from build123d import *

# Parameters (mm, degrees)
PAD005_DEPTH    = 50
SKETCH012_R     = 2.1
POCKET004_DEPTH = 50.001
POCKET005_DEPTH = 8
SKETCH014_W     = 7.2
SKETCH014_H     = 3.4
POCKET006_DEPTH = 8.85
SKETCH015_R     = 1.45
POCKET007_DEPTH = 21.801
FILLET012_R     = 3
FILLET013_R     = 3
FILLET015_R     = 1


with BuildPart() as part:
    # Sketch010 → Pad005 (new body)
    with BuildSketch(Plane.XZ):
        Polygon((-9.9, -11.8), (9.9, -11.8), (9.9, 0), (19.1, 0), (19.1, 10), (-19.1, 10), (-19.1, 0), (-9.9, 0), align=None)
    extrude(amount=PAD005_DEPTH)

    # Sketch012 → Pocket004 (cut, through all)
    with BuildSketch(Plane.XZ):
        with Locations((0, -7)):
            Circle(SKETCH012_R)
    extrude(amount=POCKET004_DEPTH, mode=Mode.SUBTRACT)

    # Sketch013 → Pocket005 (cut, symmetric)
    with BuildSketch(Plane.YZ):
        with BuildLine():
            Line((-24.861402, 6.200002), (-36.703512, -3.006758))
            ThreePointArc((-45.296488, 8.045878), (-46.526318, -1.776928), (-36.703512, -3.006758))
            Line((-42.783017, 10), (-45.296488, 8.045878))
            Line((0, 10), (-42.783017, 10))
            Line((0.003511, 6.200002), (0, 10))
            Line((-24.861402, 6.200002), (0.003511, 6.200002))
        make_face()
        with BuildLine():
            ThreePointArc((-43.455136, 5.677456), (-44.157896, 0.064424), (-38.544864, -0.638336))
            Line((-38.544864, -0.638336), (-29.749115, 6.200002))
            Line((-42.783017, 6.200002), (-29.749115, 6.200002))
            Line((-43.455136, 5.677456), (-42.783017, 6.200002))
        make_face(mode=Mode.SUBTRACT)
    extrude(amount=POCKET005_DEPTH, both=True, mode=Mode.SUBTRACT)

    # Sketch014 (on Face1 of Pocket005) → Pocket006 (cut)
    with BuildSketch(Plane(origin=(0, 0, -11.8), x_dir=(1, 0, 0), z_dir=(0, 0, -1))):
        with Locations((0, 21.756458)):
            Rectangle(SKETCH014_W, SKETCH014_H)
    extrude(amount=-POCKET006_DEPTH, mode=Mode.SUBTRACT)

    # Sketch015 (on DatumPlane) → Pocket007 (cut, through all)
    with BuildSketch(Plane.XY.offset(10)):
        with Locations((-12.1, -7)):
            Circle(SKETCH015_R)
        with Locations((12.1, -7)):
            Circle(SKETCH015_R)
        with Locations((12.1, -43)):
            Circle(SKETCH015_R)
        with Locations((-12.1, -43)):
            Circle(SKETCH015_R)
    extrude(amount=-POCKET007_DEPTH, mode=Mode.SUBTRACT)

    # Fillet012
    fillet012_edges = [part.edges().sort_by_distance(p)[0] for p in [
        (19.1, -50, 5),
        (19.1, 0, 5),
        (-19.1, -50, 5),
        (-19.1, 0, 5),
    ]]
    fillet(fillet012_edges, radius=FILLET012_R)

    # Fillet013
    fillet013_edges = [part.edges().sort_by_distance(p)[0] for p in [
        (0, -42.783017, 6.200002),
        (0, -24.861402, 6.200002),
    ]]
    fillet(fillet013_edges, radius=FILLET013_R)

    # Fillet015
    fillet015_edges = [part.edges().sort_by_distance(p)[0] for p in [
        (0, 0, 6.200002),
    ]]
    fillet(fillet015_edges, radius=FILLET015_R)


solid = part.part
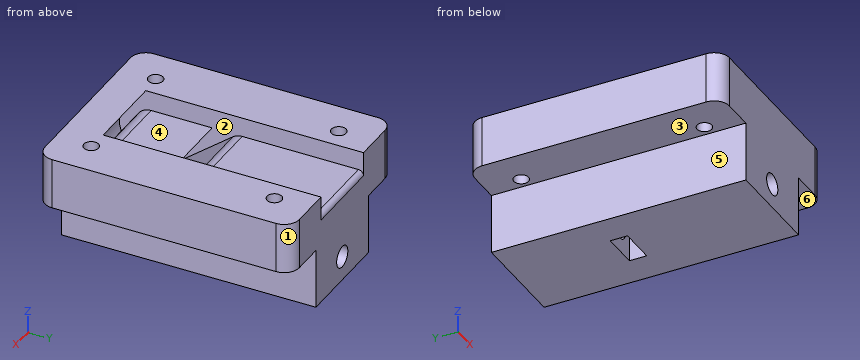
The model under review builds one solid part; all positions refer to its coordinate system, in mm. Face numbers are marked on the shaded views. A direction names the side the tool comes from. Give positions to 0.01 mm unless a question says otherwise; leave off trailing zeros. Write each loop counter-clockwise with the first axis right and the second up, starting at its lowest first coordinate (ties: lowest second). Pieces come first, ordered by that corner, then holes. Notation, with made-up numbers: M 68.25,19 L 112.25,19 A30 cw 112.25,41 Z; hole C 36,37.25 d11. An arc over 180 degrees is marked long. One line per question, with ' | ' between items. Start each with the question number.
Item 1: Draft analysis for pull direction X (two halves, no side actions). For the marked faces 1, 2 and 3, state which applies: released by +X, released by -X, zero draft, split by the parting line, or undercut.
Item 2: We need section D-D on y = -17. Write out the cut boundary in (x, z), plus the area to 3 significant figures.
Item 3: Wall thickness on line 1 (Y direction, x = -12.1, z = 5); line 2 (Z direction, x = 0, y = -6); line 3 (X direction, y = -13, z = -7): over which ranges is each line inside the solid? List them lowest first. Write a range as from..to.
Item 4: For the marked faces 4, 5 and 6, list the 3-axis set-ups (+Z, -Z, +X, -X, +Y, -Y) from which the entire face can be reached by the end or side of a thin tool; tool diameter is ignored.
Item 5: For pin 1 (5.5 mm diameter, centred on x = 0, z = -7, fed in from -Y); pin 2 (1.5 mm diameter, centred on x = 12.5, y = -26, fed in from -Z); pin 3 (6 mm diameter, centred on x = -15, z = -6.5, fed in from -Y); pin 4 (6 mm diameter, centred on y = -28, z = -5, fed in from +X), all flat-tipped, find the tip position at first contact; note any pin that passes through.
Item 6: We need section B-B on x = 12.1. Write out the cut boundary in (y, z), plus the area to 3 significant figures.
Item 7: We need section A-A on y = -7. Write out the cut boundary in (x, z), plus the area to 3 significant figures.
Item 8: We need section C-C on z = -7. Write out the cut boundary in (x, y), plus the area to 3 significant figures.
Results found:
1) face 1: released by +X | face 2: undercut | face 3: zero draft
2) outline: M -19.1,0 L -9.9,0 L -9.9,-11.8 L 9.9,-11.8 L 9.9,0 L 19.1,0 L 19.1,10 L 8,10 L 8,6.2 L -8,6.2 L -8,10 L -19.1,10 Z; hole C 0,-7 d4.2 | area: 541 mm2
3) line 1: y = -50..-44.45, -41.55..-8.45, -5.55..0 | line 2: z = -11.8..-9.1, -4.9..6.2 | line 3: x = -9.9..-2.1, 2.1..9.9
4) face 4: +Z, +Y | face 5: -Z, -X, +Y, -Y | face 6: -Z, +X, +Y, -Y
5) pin 1: stops at y = -50 | pin 2: stops at z = 0 | pin 3: passes through | pin 4: stops at x = 9.9
6) outline: M -50,0 L -44.45,0 L -44.45,10 L -50,10 Z; M -41.55,0 L -8.45,0 L -8.45,10 L -41.55,10 Z; M -5.55,0 L 0,0 L 0,10 L -5.55,10 Z | area: 442 mm2
7) outline: M -19.1,0 L -13.55,0 L -13.55,10 L -19.1,10 Z; M -10.65,0 L -9.9,0 L -9.9,-11.8 L 9.9,-11.8 L 9.9,0 L 10.65,0 L 10.65,10 L 8,10 L 8,6.2 L -8,6.2 L -8,10 L -10.65,10 Z; M 13.55,0 L 19.1,0 L 19.1,10 L 13.55,10 Z; hole C 0,-7 d4.2 | area: 483 mm2
8) outline: M -9.9,-50 L -2.1,-50 L -2.1,-23.46 L -3.6,-23.46 L -3.6,-20.06 L -2.1,-20.06 L -2.1,0 L -9.9,0 Z; M 2.1,-50 L 9.9,-50 L 9.9,0 L 2.1,0 L 2.1,-20.06 L 3.6,-20.06 L 3.6,-23.46 L 2.1,-23.46 Z | area: 770 mm2
